from build123d import *

# Parameters (mm, degrees)
SKETCH1_R                = 15
BOSS_EXTRUDE1_DEPTH      = 5
SKETCH2_R                = 12
SKETCH2_R_2              = 6.302
SKETCH2_R_3              = 3.302
CUT_EXTRUDE1_DEPTH       = 22.794494718
SKETCH4_R                = 1.55
BOSS_EXTRUDE2_DEPTH      = 7
BOSS_EXTRUDE2_2_DEPTH    = 7
BOSS_EXTRUDE2_3_DEPTH    = 7
BOSS_EXTRUDE2_4_DEPTH    = 7
BOSS_EXTRUDE2_5_DEPTH    = 7
BOSS_EXTRUDE2_6_DEPTH    = 7
SKETCH5_W                = 2.5
SKETCH5_H                = 8.771038414
BOSS_EXTRUDE3_DEPTH      = 5
CIRPATTERN1_COUNT        = 6
SKETCH6_R                = 15
SKETCH6_R_2              = 13.5
BOSS_EXTRUDE4_DEPTH      = 1.75
SKETCH7_R                = 3.25
SKETCH7_R_2              = 1.5
BOSS_EXTRUDE5_DEPTH      = 6.75
FILLET2_R                = 5
CIRPATTERN2_COUNT        = 3
FILLET2_OF_CIRPATTERN2_R = 5


with BuildPart() as part:
    # Sketch1 → Boss-Extrude1 (new body)
    with BuildSketch(Plane.XY):
        Circle(SKETCH1_R)
    extrude(amount=BOSS_EXTRUDE1_DEPTH)

    # Sketch2 → Cut-Extrude1 (cut, through all)
    with BuildSketch(Plane.XY.offset(5)):
        Circle(SKETCH2_R)
        Circle(SKETCH2_R_2, mode=Mode.SUBTRACT)
        Circle(SKETCH2_R_3)
    extrude(amount=-CUT_EXTRUDE1_DEPTH, mode=Mode.SUBTRACT)


with BuildPart() as cut_extrude1_piece_1:
    # of the separate pieces the step leaves, piece 1, a body of its own (cut_extrude1_pieces)
    add(part.part.solids().sort_by_distance((15, 0, 0))[0])



with BuildPart() as cut_extrude1_piece_2:
    # of the separate pieces the step leaves, piece 2, a body of its own (cut_extrude1_pieces)
    add(part.part.solids().sort_by_distance((6.302, 0, 0))[0])


with BuildPart() as body_3:
    # Sketch4 → Boss-Extrude2 (new body)
    with BuildSketch(Plane.XY):
        with Locations((0, 10)):
            Circle(SKETCH4_R)
    extrude(amount=BOSS_EXTRUDE2_DEPTH)


with BuildPart() as body_4:
    # Sketch4 → Boss-Extrude2 2 (new body)
    with BuildSketch(Plane.XY):
        with Locations((-8.660254038, 5)):
            Circle(SKETCH4_R)
    extrude(amount=BOSS_EXTRUDE2_2_DEPTH)


with BuildPart() as body_5:
    # Sketch4 → Boss-Extrude2 3 (new body)
    with BuildSketch(Plane.XY):
        with Locations((-8.660254038, -5)):
            Circle(SKETCH4_R)
    extrude(amount=BOSS_EXTRUDE2_3_DEPTH)


with BuildPart() as body_6:
    # Sketch4 → Boss-Extrude2 4 (new body)
    with BuildSketch(Plane.XY):
        with Locations((0, -10)):
            Circle(SKETCH4_R)
    extrude(amount=BOSS_EXTRUDE2_4_DEPTH)


with BuildPart() as body_7:
    # Sketch4 → Boss-Extrude2 5 (new body)
    with BuildSketch(Plane.XY):
        with Locations((8.660254038, -5)):
            Circle(SKETCH4_R)
    extrude(amount=BOSS_EXTRUDE2_5_DEPTH)


with BuildPart() as body_8:
    # Sketch4 → Boss-Extrude2 6 (new body)
    with BuildSketch(Plane.XY):
        with Locations((8.660254038, 5)):
            Circle(SKETCH4_R)
    extrude(amount=BOSS_EXTRUDE2_6_DEPTH)



with BuildPart() as cut_extrude1_piece_1_1:
    add(cut_extrude1_piece_1.part)

    add(cut_extrude1_piece_2.part)  # Boss-Extrude3 merges Cut-Extrude1 piece 2
    # Sketch5 → Boss-Extrude3 (add)
    with BuildSketch(Plane(origin=(0, 0, 0), x_dir=(-1, 0, 0), z_dir=(0, 0, -1))):
        with Locations((0, 10.562306722)):
            Rectangle(SKETCH5_W, SKETCH5_H)
    boss_extrude3 = extrude(amount=-BOSS_EXTRUDE3_DEPTH)

    # CirPattern1: Boss-Extrude3 ×6 about axis
    cirpattern1_axis = Axis((0, 0, 0), (0, 0, 1))
    for i in range(1, CIRPATTERN1_COUNT):
        add(boss_extrude3.rotate(cirpattern1_axis, i * 360 / CIRPATTERN1_COUNT))


with BuildPart() as body_8_1:
    add(body_8.part)

    add(cut_extrude1_piece_1_1.part)  # Boss-Extrude4 merges Cut-Extrude1 piece 1

    add(body_3.part)  # Boss-Extrude4 merges body 3

    add(body_4.part)  # Boss-Extrude4 merges body 4

    add(body_5.part)  # Boss-Extrude4 merges body 5

    add(body_6.part)  # Boss-Extrude4 merges body 6

    add(body_7.part)  # Boss-Extrude4 merges body 7
    # Sketch6 → Boss-Extrude4 (add)
    with BuildSketch(Plane.XY.offset(5)):
        Circle(SKETCH6_R)
        Circle(SKETCH6_R_2, mode=Mode.SUBTRACT)
    extrude(amount=BOSS_EXTRUDE4_DEPTH)

    # Sketch7 → Boss-Extrude5 (add)
    with BuildSketch(Plane(origin=(0, 0, 0), x_dir=(-1, 0, 0), z_dir=(0, 0, -1))):
        with Locations((0, 17.25)):
            Circle(SKETCH7_R)
        with Locations((0, 17.25)):
            Circle(SKETCH7_R_2, mode=Mode.SUBTRACT)
    boss_extrude5 = extrude(amount=-BOSS_EXTRUDE5_DEPTH)

    # Fillet2
    fillet2_edges = [body_8_1.edges().sort_by_distance(p)[0] for p in [
        (2.181099234, 14.84057971, 3.375),
        (-2.181099234, 14.84057971, 3.375),
    ]]
    fillet(fillet2_edges, radius=FILLET2_R)

    # CirPattern2: Boss-Extrude5 ×3 about axis
    cirpattern2_axis = Axis((0, 0, 0), (0, 0, 1))
    for i in range(1, CIRPATTERN2_COUNT):
        add(boss_extrude5.rotate(cirpattern2_axis, i * 360 / CIRPATTERN2_COUNT))

    # Fillet2 of CirPattern2
    fillet2_of_cirpattern2_edges = [body_8_1.edges().sort_by_distance(p)[0] for p in [
        (-13.942868653, -5.531402511, 3.375),
        (-11.761769419, -9.3091772, 3.375),
        (11.761769419, -9.3091772, 3.375),
        (13.942868653, -5.531402511, 3.375),
    ]]
    fillet(fillet2_of_cirpattern2_edges, radius=FILLET2_OF_CIRPATTERN2_R)


solid = body_8_1.part
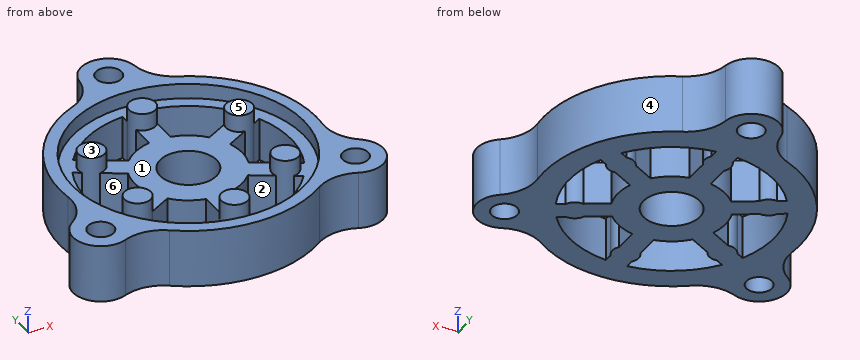
Source: CAD feature listing. Evaluate the final solid. Frame: model axes, mm. Face numbers are marked on the shaded views. A direction names the side the tool comes from. Round coordinates to 2 decimals unless told otherwise and drop trailing zeros. Loops run counter-clockwise (first coordinate to the right, second up) from the corner with the lowest first, then second, coordinate; pieces in that order, holes last. Notation, with made-up numbers: (83.25, 17) -> (135.25, 17) arc R13 cw to (135.25, 40) -> close; hole circle Ø3 at (-12, 10). An arc over 180 degrees is marked (long way). Answer as a JSON object with one key per item and string values. Group by question number.
Q1. Section query C-C (y = -8). Output: boundary loops of the cut face in (x, z), plus the area to 3 significant figures.
Q2. Section query D-D (y = 8). Output: boundary loops of the cut face in (x, z).
Q3. Section query A-A (y = 0). Output: boundary loops of the cut face in (x, z).
Q4. Section query B-B (x = 0). Output: boundary loops of the cut face in (y, z), plus the area to 3 significant figures.
Q5. Ray query, line 1 (Y direction, x = -6.5, z = 2.75); line 2 (X direction, y = -7.5, z = 3.25); line 3 (X direction, y = 4, z = 4.25). Return the intervals inside material, ascending. Write a range as from..to.
Q6. Mould query, pull axis X, two halves, no side actions, for the marked faces 4, 5 and 6. Classes: pulls with the +X half, pulls with the -X half, needs draft (parallel to the pull), parting line crosses it, or undercut.
Q7. Contact query for flat-ended pins moving along their axis: P1, Ø1.5, axis at y = -7, z = 2, coming from the -X side; P2, Ø0.5, axis at y = -11.5, z = 1.5, coming from the -X side; P3, Ø2.5, axis at x = 14.94, y = -8.63, coming from the -Z side; P4, Ø3, axis at y = 16, z = 1.5, coming from the -X side. Output: stop coordinate, or through.
Q8. Access query for the marked faces 1, 2 and 3. Directions: +Z, -Z, +X, -X, +Y, -Y. A direction counts if a zero-diameter tool reaches every point of the face in a straight line with its end or side. Return the directions, or none.
Completed:
{
 "1": {"outline": "(-18.13, 0) -> (-16.3, 0) -> (-16.3, 6.75) -> (-18.13, 6.75) -> close; (-13.58, 0) -> (-8.94, 0) -> (-8.94, 5) -> (-10.87, 5) -> (-10.87, 6.75) -> (-13.58, 6.75) -> close; (-1.25, 0) -> (1.25, 0) -> (1.25, 5) -> (-1.25, 5) -> close; (8.94, 0) -> (13.58, 0) -> (13.58, 6.75) -> (10.87, 6.75) -> (10.87, 5) -> (8.94, 5) -> close; (16.3, 0) -> (18.13, 0) -> (18.13, 6.75) -> (16.3, 6.75) -> close", "area": "92.9 mm²"},
 "2": {"outline": "(-12.69, 0) -> (-8.94, 0) -> (-8.94, 5) -> (-10.87, 5) -> (-10.87, 6.75) -> (-12.69, 6.75) -> close; (-1.25, 0) -> (1.25, 0) -> (1.25, 5) -> (-1.25, 5) -> close; (8.94, 0) -> (12.69, 0) -> (12.69, 6.75) -> (10.87, 6.75) -> (10.87, 5) -> (8.94, 5) -> close"},
 "3": {"outline": "(-15, 0) -> (-12, 0) -> (-12, 5) -> (-13.5, 5) -> (-13.5, 6.75) -> (-15, 6.75) -> close; (-6.3, 0) -> (-3.3, 0) -> (-3.3, 5) -> (-6.3, 5) -> close; (3.3, 0) -> (6.3, 0) -> (6.3, 5) -> (3.3, 5) -> close; (12, 0) -> (15, 0) -> (15, 6.75) -> (13.5, 6.75) -> (13.5, 5) -> (12, 5) -> close"},
 "4": {"outline": "(-15, 0) -> (-3.3, 0) -> (-3.3, 5) -> (-8.45, 5) -> (-8.45, 7) -> (-11.55, 7) -> (-11.55, 5) -> (-13.5, 5) -> (-13.5, 6.75) -> (-15, 6.75) -> close; (3.3, 0) -> (15.75, 0) -> (15.75, 6.75) -> (13.5, 6.75) -> (13.5, 5) -> (11.55, 5) -> (11.55, 7) -> (8.45, 7) -> (8.45, 5) -> (3.3, 5) -> close; (18.75, 0) -> (20.5, 0) -> (20.5, 6.75) -> (18.75, 6.75) -> close", "area": "152 mm²"},
 "5": {"line 1": "-13.52..-10.09, -5.2..-2.31, 2.31..5.2, 10.09..13.52", "line 2": "-17.99..-15.93, -13.95..-9.37, -1.25..1.25, 9.37..13.95, 15.93..17.99", "line 3": "-14.46..-11.31, -9.84..9.84, 11.31..14.46"},
 "6": {"face 4": "pulls with the +X half", "face 5": "needs draft", "face 6": "undercut"},
 "7": {"P1": "x = -18.07", "P2": "x = -16.86", "P3": "through", "P4": "x = -4.88"},
 "8": {"face 1": "+Z", "face 2": "+Z, -Z", "face 3": "+Z, +X, -X, +Y, -Y"}
}
